Here's how the part is built. I have some questions about the finished solid (model axes, mm). A direction names the side the tool comes from. Give positions to 0.01 mm unless a question says otherwise; leave off trailing zeros. Write each loop counter-clockwise with the first axis right and the second up, starting at its lowest first coordinate (ties: lowest second). Pieces come first, ordered by that corner, then holes. Notation, with made-up numbers: (-39, 78.25) -> (-27, 78.25) arc R31 ccw to (-27, 106.25) -> close; hole circle Ø9 at (-26.75, 16.5). An arc over 180 degrees is marked (long way). Return JSON: item names as keys, results as strings.
from build123d import *

# Parameters (mm, degrees)
F1_DEPTH = 63.5
F3_DEPTH = 124.46


# Not quite as in the source:
# - a pattern or mirror of a feature is missing from the dataset's text; its kind, count and spacing are read off the source's solid


with BuildPart() as f1:
    # F0 (on Front) → F1 (new body, symmetric)
    with BuildSketch(Plane.XZ):
        with BuildLine():
            ThreePointArc((-6.0325, 0), (0, 6.0325), (6.0325, 0))
            Line((6.0325, 0), (8.255, 0))
            ThreePointArc((8.255, 0), (0, 8.255), (-8.255, 0))
            Line((-8.255, 0), (-6.0325, 0))
        make_face()
    extrude(amount=F1_DEPTH, both=True)

    # F2 (on face) → F3 (join)
    with BuildSketch(Plane.XZ.offset(63.5)):
        Polygon((-6.7945, 0), (-7.493, 0), (-7.493, -1.4224), (-8.128, -1.4224), (-8.128, -2.6162), (-6.1595, -2.6162), (-6.1595, -1.4224), (-6.7945, -1.4224), align=None)
    f3 = extrude(amount=-F3_DEPTH)

    # F3_copies: F3 across plane
    add(f3.mirror(Plane(origin=(0, 0, 0), x_dir=(0, 0, 1), z_dir=(1, 0, 0))))


solid = f1.part
1. Suppose I cut it at B-B, the plane z = 3.5. List the corners of the cut face in (x, y) for me, and give its area (3 significant figures).
Taken from the geometry:
{"outline": "(-7.48, -63.5) -> (-4.91, -63.5) -> (-4.91, 63.5) -> (-7.48, 63.5) -> close; (4.91, -63.5) -> (7.48, -63.5) -> (7.48, 63.5) -> (4.91, 63.5) -> close", "area": "651 mm²"}
2. Suppose I cut it at C-C, the plane x = 0. List the corners of the cut face in (y, z) for me (1 decimal).
Taken from the geometry:
{"outline": "(-63.5, 6) -> (63.5, 6) -> (63.5, 8.3) -> (-63.5, 8.3) -> close"}
3. For pin 1 Ø0.5 at (x, y) = (-6.5, 3.5) entering from +Z; pin 2 Ø0.6 at (x, z) = (7.5, -2) entering from +Y; pin 3 Ø0.6 at (y, z) = (-13.5, -2) entering from -X, each with a flat end and sliding along its axis, tell me the tip position at first contact or that it passes through.
Taken from the geometry:
{"pin 1": "stops at z = 5.39", "pin 2": "stops at y = 60.96", "pin 3": "stops at x = -8.13"}
4. Which directions (+Z, -Z, +X, -X, +Y, -Y) give clear straight access to the entire face, cutting with the end or side of a thin tool? Please do faces 1 (the face through (7, 60.96, -2)), 2 (the face through (7, -2, -2.616)).
Taken from the geometry:
{"face 1": "-Z, +X, -X, +Y", "face 2": "-Z, +X, -X, +Y, -Y"}
5. Suppose I cut it at A-A, the plane y = -29. List the corners of the cut face in (x, z) for me (1 decimal).
Taken from the geometry:
{"outline": "(-8.3, 0) -> (-7.5, 0) -> (-7.5, -1.4) -> (-8.1, -1.4) -> (-8.1, -2.6) -> (-6.2, -2.6) -> (-6.2, -1.4) -> (-6.8, -1.4) -> (-6.8, 0) -> (-6, 0) arc R6 cw to (6, 0) -> (6.8, 0) -> (6.8, -1.4) -> (6.2, -1.4) -> (6.2, -2.6) -> (8.1, -2.6) -> (8.1, -1.4) -> (7.5, -1.4) -> (7.5, 0) -> (8.3, 0) arc R8.3 ccw to start"}
6. If we mould it in two halves opening along Z, with no side actions, what happens to faces 3 (the face through (-8, -1, 0)), 4 (the face through (0.182, -0.889, 8.253)), 5 (the face through (6.6, -0.9, 0)), 6 (the face through (-7, -2, -2.616))? For each: released by +Z, released by -Z, zero draft, split by the parting line, or undercut.
Taken from the geometry:
{"face 3": "undercut", "face 4": "released by +Z", "face 5": "undercut", "face 6": "released by -Z"}
7. If I drill on line 1 (X direction, y = -47, z = -1.25); line 2 (X direction, y = -23, z = -1.5); line 3 (Z direction, x = 0, y = 4) (1 decimal), over which ranges is the centre line in solid material (lowest first)? Write a range as [from, to].
Taken from the geometry:
{"line 1": "x = [-7.49, -6.79], [6.79, 7.49]", "line 2": "x = [-8.13, -6.16], [6.16, 8.13]", "line 3": "z = [6, 8.3]"}
